```python
from build123d import *

# Parameters (mm, degrees)
SKETCH1_R           = 17
SKETCH1_R_2         = 2
SKETCH1_R_3         = 8
BOSS_EXTRUDE1_DEPTH = 4
SKETCH2_R           = 2.75
SKETCH2_R_2         = 2
BOSS_EXTRUDE2_DEPTH = 3


with BuildPart() as part:
    # Sketch1 → Boss-Extrude1 (new body)
    with BuildSketch(Plane(origin=(0, 0, 0), x_dir=(0, 0, -1), z_dir=(1, 0, 0))):
        Circle(SKETCH1_R)
        with Locations((0, 12)):
            Circle(SKETCH1_R_2, mode=Mode.SUBTRACT)
        with Locations((8.485281374, 8.485281374)):
            Circle(SKETCH1_R_2, mode=Mode.SUBTRACT)
        with Locations((12, 0)):
            Circle(SKETCH1_R_2, mode=Mode.SUBTRACT)
        with Locations((8.485281374, -8.485281374)):
            Circle(SKETCH1_R_2, mode=Mode.SUBTRACT)
        with Locations((0, -12)):
            Circle(SKETCH1_R_2, mode=Mode.SUBTRACT)
        with Locations((-8.485281374, -8.485281374)):
            Circle(SKETCH1_R_2, mode=Mode.SUBTRACT)
        with Locations((-12, 0)):
            Circle(SKETCH1_R_2, mode=Mode.SUBTRACT)
        with Locations((-8.485281374, 8.485281374)):
            Circle(SKETCH1_R_2, mode=Mode.SUBTRACT)
        Circle(SKETCH1_R_3, mode=Mode.SUBTRACT)
    extrude(amount=BOSS_EXTRUDE1_DEPTH)

    # Sketch2 → Boss-Extrude2 (add)
    # profile 1 of 8: a face of its own
    with BuildSketch(Plane(origin=(4, 0, 0), x_dir=(0, 0, -1), z_dir=(1, 0, 0))):
        with Locations((8.485281374, 8.485281374)):
            Circle(SKETCH2_R)
        with Locations((8.485281374, 8.485281374)):
            Circle(SKETCH2_R_2, mode=Mode.SUBTRACT)
    # profile 2 of 8: a face of its own
    with BuildSketch(Plane(origin=(4, 0, 0), x_dir=(0, 0, -1), z_dir=(1, 0, 0))):
        with Locations((12, 0)):
            Circle(SKETCH2_R)
        with Locations((12, 0)):
            Circle(SKETCH2_R_2, mode=Mode.SUBTRACT)
    # profile 3 of 8: a face of its own
    with BuildSketch(Plane(origin=(4, 0, 0), x_dir=(0, 0, -1), z_dir=(1, 0, 0))):
        with Locations((8.485281374, -8.485281374)):
            Circle(SKETCH2_R)
        with Locations((8.485281374, -8.485281374)):
            Circle(SKETCH2_R_2, mode=Mode.SUBTRACT)
    # profile 4 of 8: a face of its own
    with BuildSketch(Plane(origin=(4, 0, 0), x_dir=(0, 0, -1), z_dir=(1, 0, 0))):
        with Locations((0, -12)):
            Circle(SKETCH2_R)
        with Locations((0, -12)):
            Circle(SKETCH2_R_2, mode=Mode.SUBTRACT)
    # profile 5 of 8: a face of its own
    with BuildSketch(Plane(origin=(4, 0, 0), x_dir=(0, 0, -1), z_dir=(1, 0, 0))):
        with Locations((-8.485281374, -8.485281374)):
            Circle(SKETCH2_R)
        with Locations((-8.485281374, -8.485281374)):
            Circle(SKETCH2_R_2, mode=Mode.SUBTRACT)
    # profile 6 of 8: a face of its own
    with BuildSketch(Plane(origin=(4, 0, 0), x_dir=(0, 0, -1), z_dir=(1, 0, 0))):
        with Locations((-12, 0)):
            Circle(SKETCH2_R)
        with Locations((-12, 0)):
            Circle(SKETCH2_R_2, mode=Mode.SUBTRACT)
    # profile 7 of 8: a face of its own
    with BuildSketch(Plane(origin=(4, 0, 0), x_dir=(0, 0, -1), z_dir=(1, 0, 0))):
        with Locations((-8.485281374, 8.485281374)):
            Circle(SKETCH2_R)
        with Locations((-8.485281374, 8.485281374)):
            Circle(SKETCH2_R_2, mode=Mode.SUBTRACT)
    # profile 8 of 8: a face of its own
    with BuildSketch(Plane(origin=(4, 0, 0), x_dir=(0, 0, -1), z_dir=(1, 0, 0))):
        with Locations((0, 12)):
            Circle(SKETCH2_R)
        with Locations((0, 12)):
            Circle(SKETCH2_R_2, mode=Mode.SUBTRACT)
    extrude(amount=BOSS_EXTRUDE2_DEPTH)


solid = part.part
```
The model under review builds one solid part; all positions refer to its coordinate system, in mm. A direction names the side the tool comes from. Give positions to 0.01 mm unless a question says otherwise; leave off trailing zeros. Write each loop counter-clockwise with the first axis right and the second up, starting at its lowest first coordinate (ties: lowest second). Pieces come first, ordered by that corner, then holes.
(1) For P1, Ø3, axis at y = -8.49, z = 8.49, coming from the -X side; P2, Ø4, axis at x = 4.5, z = -7.5, coming from the +Y side; P3, Ø3, axis at x = 4.5, z = 4, coming from the -Y side, all flat-tipped, find the tip position at first contact; note any pin that passes through.
(2) Consider section A-A, the plane z = 0. Give the boundary of the cut face in (x, y).
(3) To check wall thickness, follow L1, parallel to Y at x = 3.5, z = 0; L2, parallel to Z at x = 0.75, y = -0.5; L3, parallel to Z at x = 6.5, y = -7. State the ranges of each line that lie inside material, in increasing order.
(4) The part is to be moulded in two halves that separate along Z. For faces 1 (the cylindrical face through (1.972, 14.334, -9.139)), 2 (the flat face through (0, 4, -7.3)), 3 (the cylindrical face through (5.479, 8.606, 11.233)), 4 (the cylindrical face through (5.48, 9.31, -11.11)), say which applies: released by +Z, released by -Z, zero draft, split by the parting line, or undercut.
(5) Consider section D-D, the plane x = 3.25. Give the number of separate pieces and of enclosed holes in the cut face, and give its area (3 significant figures).
(6) Tool access review of faces 5 (the flat face through (4, 4, -7.3)), 6 (the cylindrical face through (1.97, -7.81, 1.73)): name each direction out of +Z, -Z, +X, -X, +Y, -Y from which nothing blocks a thin tool from reaching the whole face with its end or side.
(7) Consider section B-B, the plane y = 12. Give the boundary of the cut face in (x, z), and give its area (3 significant figures).
Returned:
1. P1: passes through
1. P2: stops at y = 16.06
1. P3: stops at y = -16.8
2. outline: (0, -17) - (4, -17) - (4, -14.75) - (7, -14.75) - (7, -14) - (0, -14) - close; (0, -10) - (7, -10) - (7, -9.25) - (4, -9.25) - (4, -8) - (0, -8) - close; (0, 8) - (4, 8) - (4, 9.25) - (7, 9.25) - (7, 10) - (0, 10) - close; (0, 14) - (7, 14) - (7, 14.75) - (4, 14.75) - (4, 17) - (0, 17) - close
3. L1: y = -17 to -14, -10 to -8, 8 to 10, 14 to 17
3. L2: z = -16.99 to -13.94, -10.06 to -7.98, 7.98 to 10.06, 13.94 to 16.99
3. L3: z = -10.8 to -9.82, -7.15 to -6.17, 6.17 to 7.15, 9.82 to 10.8
4. face 1: split by the parting line
4. face 2: zero draft
4. face 3: undercut
4. face 4: undercut
5. separate pieces: 1
5. enclosed holes: 9
5. area: 606 mm2
6. face 5: +X
6. face 6: +X, -X
7. outline: (0, -12.04) - (4, -12.04) - (4, -2.75) - (7, -2.75) - (7, -2) - (0, -2) - close; (0, 2) - (7, 2) - (7, 2.75) - (4, 2.75) - (4, 12.04) - (0, 12.04) - close
7. area: 84.8 mm2
